Part model, mm, in its own coordinate system. A direction names the side the tool comes from. Round coordinates to 2 decimals unless told otherwise and drop trailing zeros. Order: outer loops, then holes, each group sorted by start corner. A loop starts at its lowest first (then second) coordinate and runs counter-clockwise, first axis right, second up. Notation, with made-up numbers: (55, 79.25) - (96, 79.25) arc R19 cw to (96, 107.25) - close; hole circle Ø11 at (-37.75, -22.75). An arc over 180 degrees is marked (long way). Return JSON: item names as keys, results as strings. Group by question number.
Item 1: Drop flat-ended pins along their axis: pin 1 (12.5 mm diameter, centred on x = 53.34, y = 101.6, fed in from +Z) (3 decimals); pin 2 (3 mm diameter, centred on y = -7.5, z = 82.5, fed in from +X) (3 decimals). Give the stop position or say it passes through.
Item 2: Saw through at D-D on y = 101.6. List the corners of the cut face in (x, z) (3 decimals).
Item 3: Probe probe 1 along Y at (x, z) = (53.34, 4.5); probe 2 along X at (y, z) = (-101, 5); probe 3 along Z at (x, y) = (35, 85.5) (3 decimals). List the from-to ranges inside material, lowest first.
Item 4: Saw through at C-C on y = -67. List the corners of the cut face in (x, z) (3 decimals).
Item 5: Two-plate mould, pull along Z, no slides. Class faces 1 (the face through (100.07, -1.78, 8.08)), 2 (the face through (9, 127, 36)), 3 (the face through (5, 90.488, 63)): released by +Z, released by -Z, zero draft, split by the parting line, or undercut.
Item 6: Tool access for faces 4 (the face through (101.6, -2, 2)), 5 (the face through (9.525, -2, 55)), 6 (the face through (4.696, -98.6, 79.102)): list every direction of +Z, -Z, +X, -X, +Y, -Y with a clear straight run to the whole face (end or side of a thin tool).
Item 7: Saw through at B-B on x = 53.34. List the corners of the cut face in (y, z) (3 decimals).
Item 8: Saw through at A-A on z = 61.5. List the corners of the cut face in (x, y) (1 decimal).
```python
from build123d import *

# Parameters (mm, degrees)
F1_DEPTH = 127
F2_R     = 5.08
F4_DEPTH = 25.4
F5_R     = 3.96875
F6_DEPTH = 25.4


with BuildPart() as f1:
    # F0 (on Front) → F1 (new body, symmetric)
    with BuildSketch(Plane.XZ):
        Polygon((0, 101.6), (0, 0), (101.6, 0), (101.6, 9.525), (9.525, 9.525), (9.525, 101.6), align=None)
    extrude(amount=F1_DEPTH, both=True)

    # F2
    f2_edges = [f1.edges().sort_by_distance(p)[0] for p in [
        (9.525, 0, 9.525),
        (0, 0, 0),
        (9.525, 0, 101.6),
        (101.6, 0, 9.525),
    ]]
    fillet(f2_edges, radius=F2_R)

    # F3 (on face) → F4 (cut)
    with BuildSketch(Plane(origin=(0, 0, 0), x_dir=(0, -1, 0), z_dir=(-1, 0, 0))):
        with BuildLine():
            Line((-90.4875, 55.614824), (-90.4875, 71.166491))
            ThreePointArc((-90.4875, 71.166491), (-98.425, 79.103991), (-106.3625, 71.166491))
            Line((-106.3625, 71.166491), (-106.3625, 55.614824))
            ThreePointArc((-106.3625, 55.614824), (-98.425, 47.677324), (-90.4875, 55.614824))
        make_face()
        with BuildLine():
            ThreePointArc((90.4875, 55.614824), (98.425, 47.677324), (106.3625, 55.614824))
            Line((106.3625, 55.614824), (106.3625, 71.166491))
            ThreePointArc((106.3625, 71.166491), (98.425, 79.103991), (90.4875, 71.166491))
            Line((90.4875, 71.166491), (90.4875, 55.614824))
        make_face()
    extrude(amount=-F4_DEPTH, mode=Mode.SUBTRACT)

    # F5 (on face) → F6 (cut)
    with BuildSketch(Plane(origin=(0, 0, 0), x_dir=(1, 0, 0), z_dir=(0, 0, -1))):
        with Locations((53.34, 101.6)):
            Circle(F5_R)
        with Locations((53.34, -101.6)):
            Circle(F5_R)
    extrude(amount=-F6_DEPTH, mode=Mode.SUBTRACT)


solid = f1.part
```
Filled in:
{
 "1": {"pin 1": "stops at z = 9.525", "pin 2": "stops at x = 9.525"},
 "2": {"outline": "(0, 5.08) arc R5.08 ccw to (5.08, 0) - (49.371, 0) - (49.371, 9.525) - (14.605, 9.525) arc R5.08 cw to (9.525, 14.605) - (9.525, 48.34) - (0, 48.34) - close; (0, 78.441) - (9.525, 78.441) - (9.525, 96.52) arc R5.08 ccw to (4.445, 101.6) - (0, 101.6) - close; (57.309, 0) - (101.6, 0) - (101.6, 4.445) arc R5.08 ccw to (96.52, 9.525) - (57.309, 9.525) - close"},
 "3": {"probe 1": "y = -127 to -105.57, -97.63 to 97.63, 105.57 to 127", "probe 2": "x = 0 to 49.42, 57.26 to 101.57", "probe 3": "z = 0 to 9.525"},
 "4": {"outline": "(0, 5.08) arc R5.08 ccw to (5.08, 0) - (101.6, 0) - (101.6, 4.445) arc R5.08 ccw to (96.52, 9.525) - (14.605, 9.525) arc R5.08 cw to (9.525, 14.605) - (9.525, 96.52) arc R5.08 ccw to (4.445, 101.6) - (0, 101.6) - close"},
 "5": {"face 1": "released by +Z", "face 2": "zero draft", "face 3": "undercut"},
 "6": {"face 4": "+Z, -Z, +X, +Y, -Y", "face 5": "+Z, +X, +Y, -Y", "face 6": "+X, -X"},
 "7": {"outline": "(-127, 0) - (-105.569, 0) - (-105.569, 9.525) - (-127, 9.525) - close; (-97.631, 0) - (97.631, 0) - (97.631, 9.525) - (-97.631, 9.525) - close; (105.569, 0) - (127, 0) - (127, 9.525) - (105.569, 9.525) - close"},
 "8": {"outline": "(0, -127) - (9.5, -127) - (9.5, -106.4) - (0, -106.4) - close; (0, -90.5) - (9.5, -90.5) - (9.5, 90.5) - (0, 90.5) - close; (0, 106.4) - (9.5, 106.4) - (9.5, 127) - (0, 127) - close"}
}
